Source: three-view drawing plus pictorial views. Frame: mm from the lowest corner of the part. A direction names the side the tool comes from. Coordinates: 2 decimals unless noted, no trailing zeros. Order: outer loops, then holes, each group sorted by start corner. A loop starts at its lowest first (then second) coordinate and runs counter-clockwise, first axis right, second up. Notation, with made-up numbers: M -23,73 L -6,73 A10 ccw -6,85 Z; hole C -27.5,80.25 d1. An arc over 180 degrees is marked long. One line per question, with ' | ' between items.
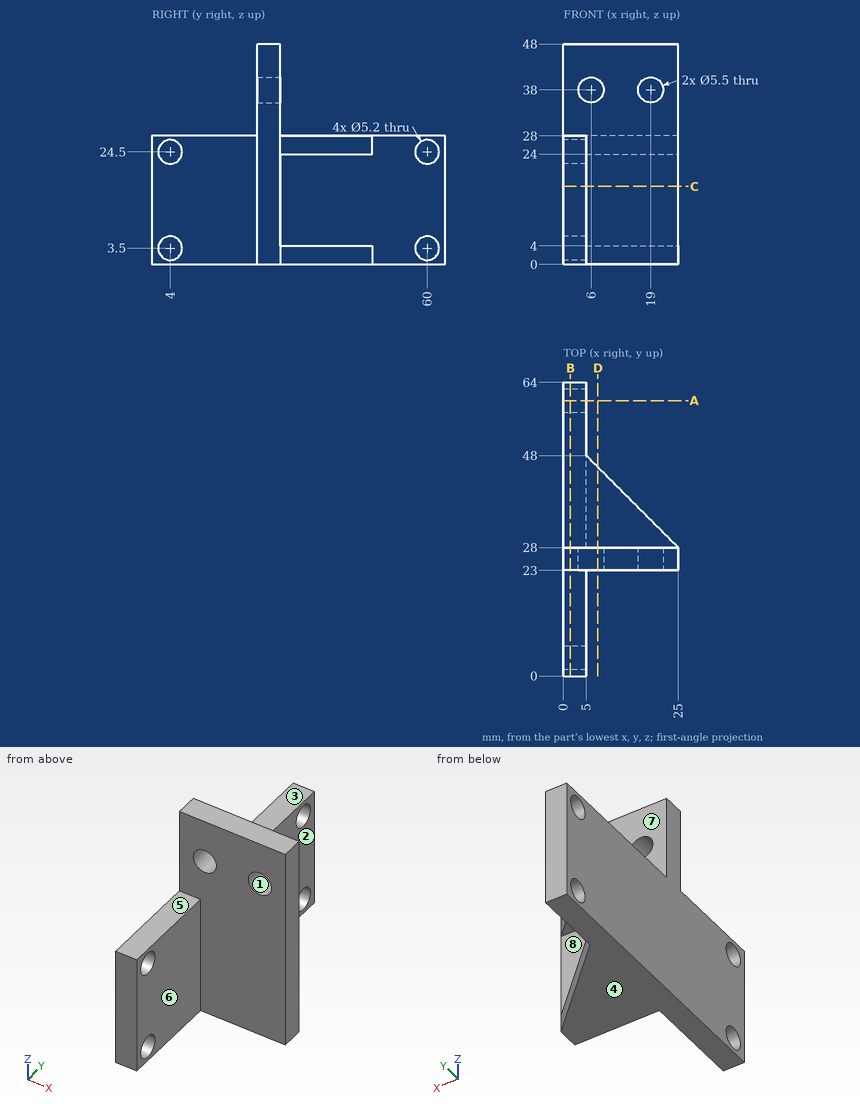
1. Draft query along X for the marked faces 1, 2 and 3. Return one class per face: pulls with the +X half, pulls with the -X half, needs draft (parallel to the pull), parting line crosses it, or undercut.
Response values:
face 1: undercut | face 2: pulls with the +X half | face 3: needs draft
2. Section C-C, the plane z = 17. Output: boundary loops of the cut face in (x, y), and give its area (3 significant figures).
Response values:
outline: M 0,0 L 5,0 L 5,23 L 25,23 L 25,28 L 5,28 L 5,64 L 0,64 Z | area: 420 mm^2
3. Access query for the marked faces 4, 5, 6, 7 and 8. Directions: +Z, -Z, +X, -X, +Y, -Y. A direction counts if a zero-diameter tool reaches every point of the face in a straight line with its end or side. Return the directions, or none.
Response values:
face 4: -Z, +X, -X, +Y, -Y | face 5: +Z, +X, -X, -Y | face 6: +Z, -Z, +X, -Y | face 7: +Z, +X, -X, +Y | face 8: +X, +Y
4. Material intervals for line 1 (Z direction, x = 2.15, y = 60); line 2 (Z direction, x = 6, y = 26.7); line 3 (Z direction, x = 19.75, y = 30), sorted ascending. Write a range as [from, to].
Response values:
line 1: z = [0, 0.9], [6.1, 21.9], [27.1, 28] | line 2: z = [0, 35.25], [40.75, 48] | line 3: z = [0, 4], [24, 28]
5. Section A-A, the plane y = 60. Output: boundary loops of the cut face in (x, z).
Response values:
outline: M 0,0 L 5,0 L 5,0.9 L 0,0.9 Z; M 0,6.1 L 5,6.1 L 5,21.9 L 0,21.9 Z; M 0,27.1 L 5,27.1 L 5,28 L 0,28 Z
6. Section D-D, the plane x = 7.5. Output: boundary loops of the cut face in (y, z) (1 decimal).
Response values:
outline: M 23,0 L 45.5,0 L 45.5,4 L 28,4 L 28,24 L 45.5,24 L 45.5,28 L 28,28 L 28,35.7 L 23,35.7 Z; M 23,40.3 L 28,40.3 L 28,48 L 23,48 Z
7. Pin query (flat end, axial travel): P1, Ø2.5, axis at x = 2.5, y = 12, coming from the +Z side; P2, Ø9, axis at x = 6, z = 38, coming from the +Y side; P3, Ø4, axis at x = 14.5, z = 25, coming from the -Y side; P4, Ø4, axis at y = 60, z = 24.5, coming from the +X side. Return the tip coordinate at first contact, or that it passes through.
Response values:
P1: stops at z = 28 | P2: stops at y = 28 | P3: stops at y = 23 | P4: passes through
8. Section B-B, the plane x = 1.5. Output: boundary loops of the cut face in (y, z).
Response values:
outline: M 0,0 L 64,0 L 64,28 L 28,28 L 28,48 L 23,48 L 23,28 L 0,28 Z; hole C 4,3.5 d5.2; hole C 4,24.5 d5.2; hole C 60,3.5 d5.2; hole C 60,24.5 d5.2
